from build123d import *

# Parameters (mm, degrees)
SKETCH1_W           = 24
SKETCH1_H           = 43
SKETCH1_R           = 0.45
BOSS_EXTRUDE1_DEPTH = 1.6
SKETCH2_W           = 23
SKETCH2_H           = 33.5
BOSS_EXTRUDE2_DEPTH = 2.6
FILLET1_R           = 0.3


with BuildPart() as part:
    # Sketch1 → Boss-Extrude1 (new body)
    with BuildSketch(Plane(origin=(0, 0, 0), x_dir=(1, 0, 0), z_dir=(0, 1, 0))):
        with Locations((12, 21.5)):
            Rectangle(SKETCH1_W, SKETCH1_H)
        with Locations(Location((19.62, 41.5, 0), (0, 0, 270))):
            Circle(SKETCH1_R, mode=Mode.SUBTRACT)
        with Locations(Location((17.08, 41.5, 0), (0, 0, 270))):
            Circle(SKETCH1_R, mode=Mode.SUBTRACT)
        with Locations(Location((14.54, 41.5, 0), (0, 0, 270))):
            Circle(SKETCH1_R, mode=Mode.SUBTRACT)
        with Locations(Location((12, 41.5, 0), (0, 0, 270))):
            Circle(SKETCH1_R, mode=Mode.SUBTRACT)
        with Locations(Location((9.46, 41.5, 0), (0, 0, 270))):
            Circle(SKETCH1_R, mode=Mode.SUBTRACT)
        with Locations(Location((6.92, 41.5, 0), (0, 0, 270))):
            Circle(SKETCH1_R, mode=Mode.SUBTRACT)
        with Locations(Location((4.38, 41.5, 0), (0, 0, 270))):
            Circle(SKETCH1_R, mode=Mode.SUBTRACT)
        with Locations(Location((19.8, 3, 0), (0, 0, 270))):
            Circle(SKETCH1_R, mode=Mode.SUBTRACT)
        with Locations(Location((17.26, 3, 0), (0, 0, 270))):
            Circle(SKETCH1_R, mode=Mode.SUBTRACT)
        with Locations(Location((14.72, 3, 0), (0, 0, 270))):
            Circle(SKETCH1_R, mode=Mode.SUBTRACT)
        with Locations(Location((12.18, 3, 0), (0, 0, 270))):
            Circle(SKETCH1_R, mode=Mode.SUBTRACT)
    extrude(amount=BOSS_EXTRUDE1_DEPTH)

    # Sketch2 → Boss-Extrude2 (add)
    with BuildSketch(Plane(origin=(0, 1.6, 0), x_dir=(1, 0, 0), z_dir=(0, 1, 0))):
        with Locations((12, 22.25)):
            Rectangle(SKETCH2_W, SKETCH2_H)
    extrude(amount=BOSS_EXTRUDE2_DEPTH)

    # Fillet1
    fillet1_edges = [part.edges().sort_by_distance(p)[0] for p in [
        (0.5, 4.2, -22.25),
        (12, 4.2, -5.5),
        (23.5, 4.2, -22.25),
        (12, 4.2, -39),
    ]]
    fillet(fillet1_edges, radius=FILLET1_R)


solid = part.part
CAD build for the part. Positions are in the model's coordinates, mm. A direction names the side the tool comes from. Give positions to 0.01 mm unless a question says otherwise; leave off trailing zeros. Write each loop counter-clockwise with the first axis right and the second up, starting at its lowest first coordinate (ties: lowest second). Pieces come first, ordered by that corner, then holes. Notation, with made-up numbers: M 27,15 L 71,15 A27 ccw 71,53 Z; hole C -4.75,-34 d6. An arc over 180 degrees is marked long. Put each result on its own line as item: value. Start each with the question number.
(1) Flat gauge pins, fed straight in: pin 1 Ø0.7 at (x, y) = (10, 3) entering from -Z; pin 2 Ø2.5 at (y, z) = (3, -18.5) entering from -X; pin 3 Ø1.2 at (y, z) = (2.5, -15) entering from +X. Where does each tip first touch, or does it go through?
(2) Band-saw the part on A-A, the plane z = -3. Write the cut outline in (x, y).
(3) Band-saw the part on D-D, the plane z = -8. Write the cut outline in (x, y).
(4) Probe L1, parallel to X at y = 0.9, z = -3; L2, parallel to Z at x = 17.26, y = 1.15; L3, parallel to X at y = 1.95, z = -26. List the from-to ranges inside material, lowest first.
(5) Which spindle directions (+Z, -Z, +X, -X, +Y, -Y) get a long thin tool onto all of the face, cutting with end or side? Do faces 1 (the face through (12, 3, -39)), 2 (the face through (12, 3, -5.5)), 3 (the face through (23.5, 3, -22)). Say none if no direction does.
(6) Band-saw the part on B-B, the plane x = 9.46. Write the cut outline in (y, z), and give its area (3 significant figures).
(7) Mould opens along X. For faces 4 (the face through (0.5, 3, -22)), 5 (the face through (12, 1, 0)), 6 (the face through (9.595, 0.789, -41.071)) say: +X half, -X half, draft (parallel to the pull), parting line (faces both ways), or undercut.
(8) Band-saw the part on C-C, the plane z = -41.5. Give the number of separate pieces and of enclosed holes in the cut face, and give its area (3 significant figures).
Response values:
1. pin 1: stops at z = -39
1. pin 2: stops at x = 0.5
1. pin 3: stops at x = 23.5
2. outline: M 0,0 L 11.73,0 L 11.73,1.6 L 0,1.6 Z; M 12.63,0 L 14.27,0 L 14.27,1.6 L 12.63,1.6 Z; M 15.17,0 L 16.81,0 L 16.81,1.6 L 15.17,1.6 Z; M 17.71,0 L 19.35,0 L 19.35,1.6 L 17.71,1.6 Z; M 20.25,0 L 24,0 L 24,1.6 L 20.25,1.6 Z
3. outline: M 0,0 L 24,0 L 24,1.6 L 23.5,1.6 L 23.5,3.9 A0.3 ccw 23.2,4.2 L 0.8,4.2 A0.3 ccw 0.5,3.9 L 0.5,1.6 L 0,1.6 Z
4. L1: x = 0 to 11.73, 12.63 to 14.27, 15.17 to 16.81, 17.71 to 19.35, 20.25 to 24
4. L2: z = -43 to -41.91, -41.09 to -3.45, -2.55 to 0
4. L3: x = 0.5 to 23.5
5. face 1: -Z, +X, -X, +Y
5. face 2: +Z, +X, -X, +Y
5. face 3: +Z, -Z, +X, +Y
6. outline: M 0,-43 L 1.6,-43 L 1.6,-41.95 L 0,-41.95 Z; M 0,-41.05 L 1.6,-41.05 L 1.6,-39 L 3.9,-39 A0.3 ccw 4.2,-38.7 L 4.2,-5.8 A0.3 ccw 3.9,-5.5 L 1.6,-5.5 L 1.6,0 L 0,0 Z
6. area: 154 mm2
7. face 4: -X half
7. face 5: draft
7. face 6: undercut
8. separate pieces: 8
8. enclosed holes: 0
8. area: 28.3 mm2
